```python
from build123d import *

# Parameters (mm, degrees)
SKETCH1_W           = 33.02
SKETCH1_H           = 15.24
BOSS_EXTRUDE1_DEPTH = 11.176
SKETCH2_R           = 4.7
SKETCH2_R_2         = 5.2
BOSS_EXTRUDE2_DEPTH = 5
SKETCH3_W           = 42
SKETCH3_H           = 15.24
BOSS_EXTRUDE3_DEPTH = 5


with BuildPart() as part:
    # Sketch1 → Boss-Extrude1 (new body)
    with BuildSketch(Plane(origin=(0, 0, 0), x_dir=(1, 0, 0), z_dir=(0, 1, 0))):
        Rectangle(SKETCH1_W, SKETCH1_H)
    extrude(amount=BOSS_EXTRUDE1_DEPTH)

    # Sketch2 → Boss-Extrude2 (add)
    with BuildSketch(Plane(origin=(0, 11.176, 0), x_dir=(1, 0, 0), z_dir=(0, 1, 0))):
        with Locations((-5, 0)):
            Circle(SKETCH2_R)
        with Locations((5, 0)):
            Circle(SKETCH2_R_2)
    extrude(amount=BOSS_EXTRUDE2_DEPTH)

    # Sketch3 → Boss-Extrude3 (add)
    with BuildSketch(Plane.XZ):
        Rectangle(SKETCH3_W, SKETCH3_H)
    extrude(amount=-BOSS_EXTRUDE3_DEPTH)


solid = part.part
```
CAD build for the part. Positions are in the model's coordinates, mm. A direction names the side the tool comes from. Coordinates: 2 decimals unless noted, no trailing zeros. Write each loop counter-clockwise with the first axis right and the second up, starting at its lowest first coordinate (ties: lowest second). Pieces come first, ordered by that corner, then holes. Notation, with made-up numbers: (82.5, 6.5) -> (118.5, 6.5) arc R28 ccw to (118.5, 26.5) -> close; hole circle Ø8 at (76, -29). An arc over 180 degrees is marked (long way). Return JSON: item names as keys, results as strings. Group by question number.
Q1. Cut at D-D, the plane x = 5. Give the cut face in (y, z), then the cut area to 3 significant figures.
Q2. Which spindle directions (+Z, -Z, +X, -X, +Y, -Y) get a long thin tool onto all of the face, cutting with end or side? Do faces 1 (the face through (-19, 5, 0)), 2 (the face through (0, 11.176, -2)), 3 (the face through (19, 5, 0)). Say none if no direction does.
Q3. Flat gauge pins, fed straight in: pin 1 (3 mm diameter, centred on y = 9.5, z = -3.5, fed in from -X); pin 2 (1.3 mm diameter, centred on x = 19.5, z = -1.5, fed in from +Y); pin 3 (5 mm diameter, centred on x = -18.5, z = -2, fed in from +Y). Where does each tip first touch, or does it go through?
Q4. Cut at A-A, the plane z = 0. Give the cut face in (x, y), then the cut area to 3 significant figures.
Q5. Cut at B-B, the plane x = -5. Give the cut face in (y, z).
Q6. Drill centre lines: line 1 (Y direction, x = -4, z = -6); line 2 (X direction, y = 9.25, z = -5); line 3 (X direction, y = 13.25, z = -4). Where is each one in solid material? Low to high.
Q7. Cut at C-C, the plane y = 13.25. Give the cut face in (x, z).
Q8. Pull direction X, two halves, no side cores. Call faces 4 (the face through (16.51, 8, 0)), 5 (the face through (-9.695, 13.641, -0.207)), 6 (the face through (1.167, 13.641, -3.514)), 7 (the face through (0, 6, 7.62)): released by +X, released by -X, zero draft, split by the parting line, or undercut.
Returned:
{
 "1": {"outline": "(0, -7.62) -> (11.18, -7.62) -> (11.18, -5.2) -> (16.18, -5.2) -> (16.18, 5.2) -> (11.18, 5.2) -> (11.18, 7.62) -> (0, 7.62) -> close", "area": "222 mm2"},
 "2": {"face 1": "+Z, -Z, -X, +Y", "face 2": "+Y", "face 3": "+Z, -Z, +X, +Y"},
 "3": {"pin 1": "stops at x = -16.51", "pin 2": "stops at y = 5", "pin 3": "stops at y = 11.18"},
 "4": {"outline": "(-21, 0) -> (21, 0) -> (21, 5) -> (16.51, 5) -> (16.51, 11.18) -> (10.2, 11.18) -> (10.2, 16.18) -> (-0.2, 16.18) -> (-0.2, 11.18) -> (-0.3, 11.18) -> (-0.3, 16.18) -> (-9.7, 16.18) -> (-9.7, 11.18) -> (-16.51, 11.18) -> (-16.51, 5) -> (-21, 5) -> close", "area": "513 mm2"},
 "5": {"outline": "(0, -7.62) -> (11.18, -7.62) -> (11.18, -4.7) -> (16.18, -4.7) -> (16.18, 4.7) -> (11.18, 4.7) -> (11.18, 7.62) -> (0, 7.62) -> close"},
 "6": {"line 1": "y = 0 to 11.18", "line 2": "x = -16.51 to 16.51", "line 3": "x = -7.47 to -2.53, 1.68 to 8.32"},
 "7": {"outline": "circle Ø9.4 at (-5, 0); circle Ø10.4 at (5, 0)"},
 "8": {"face 4": "released by +X", "face 5": "undercut", "face 6": "undercut", "face 7": "zero draft"}
}
